Autodesk Inventor part; units mm, degrees
ref_plane "YZ Plane" through (0, 0, 0) normal (1, 0, 0) x (0, 1, 0)
ref_plane "XZ Plane" through (0, 0, 0) normal (0, 1, 0) x (-1, 0, 0)
ref_plane "XY Plane" through (0, 0, 0) normal (0, 0, 1) x (1, 0, 0)
sketch "Sketch1" plane through (0, 0, 0) normal (0, 0, 1) x (1, 0, 0)
  line L0 (-7, -12.5) -> (7, -12.5)
  line L1 (7, -12.5) -> (7, 12.5)
  line L2 (7, 12.5) -> (-7, 12.5)
  line L3 (-7, 12.5) -> (-7, -12.5)
  line L4 (-7, -12.5) -> (7, 12.5) construction
  line L5 (7, -12.5) -> (-7, 12.5) construction
  point P0 (0, 0)
  dimension "d0" = 14
  dimension "d1" = 25
extrude "Extrusion1" add sketch "Sketch1" along normal blind 2
sketch "Sketch2" plane through (0, 0, 2) normal (0, 0, 1) x (1, 0, 0)
  circle A0 centre (0, 7.6788) radius 1.6
  line L0 (-7, 12.5) -> (-7, -12.5) construction
  line L1 (-7, 0) -> (7, 0) construction
  line L2 (7, -12.5) -> (7, 12.5) construction
  circle A1 centre (0, -7.6788) radius 1.6
  point P0 (0, 0)
  dimension "d4" = 3.2
extrude "Extrusion2" cut sketch "Sketch2" against normal blind 2
sketch "Sketch3" plane through (0, 0, 2) normal (0, 0, 1) x (1, 0, 0)
  circle A0 centre (0, 0) radius 2
  dimension "d7" = 4
extrude "Extrusion3" add sketch "Sketch3" along normal blind 10
sketch "Sketch4" plane through (0, 0, 2) normal (0, 0, 1) x (1, 0, 0)
  circle A0 centre (0, 0) radius 2
  circle A1 centre (0, 0) radius 3.5
  dimension "d10" = 1.5
extrude "Extrusion4" add sketch "Sketch4" along normal blind 2
chamfer "Chamfer1" distance 1 angle 45 2 edges at (-1.6, -7.6788, 2) (-1.6, 7.6788, 2)
properties part number "BearingMount-ExtrusionBtm"
Check sheet for the modelled part. Datum: model origin and axes. Units: mm. A direction names the side the tool comes from. Give positions to 0.01 mm unless a question says otherwise; leave off trailing zeros. Loops run counter-clockwise (first coordinate to the right, second up) from the corner with the lowest first, then second, coordinate; pieces in that order, holes last. Notation, with made-up numbers: M -17,73.5 L 17,73.5 A22 ccw 17,80.5 Z; hole C 32,0.5 d3. An arc over 180 degrees is marked long. Return JSON: item names as keys, results as strings. Group by question number.
1. Cross-section at A-A on x = 0. Record the boundary of the cut face in (y, z), plus the area to 3 significant figures.
2. Cross-section at C-C on x = 3.25. Record the boundary of the cut face in (y, z), plus the area to 3 significant figures.
3. Thickness scan on L1, parallel to Y at x = 0, z = 0.4; L2, parallel to Z at x = -2.25, y = -1; L3, parallel to Z at x = -4.5, y = 4.25. Record the ranges inside material, lowest first.
4. Tool access check on faces 4 (the cylindrical face through (3.233, 1.341, 2.986)), 5 (the flat face through (0, 12.5, 1)). Record the directions out of +Z, -Z, +X, -X, +Y, -Y that give a thin tool (end or side, any length) a straight path to the whole face; none if there is none.
5. Cross-section at D-D on z = 8.5. Record the boundary of the cut face in (x, y).
6. Cross-section at B-B on y = 0. Record the boundary of the cut face in (x, z).
7. Go/stop test with flat-tipped pins: pin 1 (2.5 mm diameter, centred on x = 0, y = 7.68, fed in from +Z); pin 2 (3 mm diameter, centred on x = 0.5, z = 5, fed in from -Y); pin 3 (2 mm diameter, centred on x = 5.5, y = 7, fed in from +Z); pin 4 (3 mm diameter, centred on y = 2.5, z = 5, fed in from +X). Record where each tip stops, or that it passes through.
8. Mould release check, pull along Y, two halves, no side actions. Record for faces 1 (the flat face through (-3, -3, 2)), 2 (the cylindrical face through (-0.208, 9.265, 0.507)), 3 (the cylindrical face through (0, 2, 8)): released by +Y, released by -Y, zero draft, split by the parting line, or undercut.
Return value:
{
 "1": {"outline": "M -12.5,0 L -9.28,0 L -9.28,1 L -10.28,2 L -12.5,2 Z; M -6.08,0 L 6.08,0 L 6.08,1 L 5.08,2 L 3.5,2 L 3.5,4 L 2,4 L 2,12 L -2,12 L -2,4 L -3.5,4 L -3.5,2 L -5.08,2 L -6.08,1 Z; M 9.28,0 L 12.5,0 L 12.5,2 L 10.28,2 L 9.28,1 Z", "area": "81.2 mm^2"},
 "2": {"outline": "M -12.5,0 L 12.5,0 L 12.5,2 L 1.3,2 L 1.3,4 L -1.3,4 L -1.3,2 L -12.5,2 Z", "area": "55.2 mm^2"},
 "3": {"L1": "-12.5 to -9.28, -6.08 to 6.08, 9.28 to 12.5", "L2": "0 to 4", "L3": "0 to 2"},
 "4": {"face 4": "+Z", "face 5": "+Z, -Z, +X, -X, +Y"},
 "5": {"outline": "C 0,0 d4"},
 "6": {"outline": "M -7,0 L 7,0 L 7,2 L 3.5,2 L 3.5,4 L 2,4 L 2,12 L -2,12 L -2,4 L -3.5,4 L -3.5,2 L -7,2 Z"},
 "7": {"pin 1": "through", "pin 2": "y = -3.5", "pin 3": "z = 2", "pin 4": "x = 3.22"},
 "8": {"face 1": "zero draft", "face 2": "undercut", "face 3": "split by the parting line"}
}
